```python
from build123d import *

# Parameters (mm, degrees)
SKETCH_W        = 70.25
SKETCH_H        = 49.7
PAD_DEPTH       = 7.1
SKETCH001_W     = 3.6
SKETCH001_H     = 9.8
SKETCH001_H_2   = 30.5
POCKET_DEPTH    = 0.9
SKETCH002_W     = 51.75
SKETCH002_H     = 5.3
PAD001_DEPTH    = 2.6
FILLET_R        = 1
SKETCH003_W     = 61.57
SKETCH003_H     = 44.62
PAD002_DEPTH    = 0.05
SKETCH004_R     = 1
POCKET001_DEPTH = 9.751


with BuildPart() as part:
    # Sketch → Pad (new body)
    with BuildSketch(Plane.XY):
        Rectangle(SKETCH_W, SKETCH_H)
    extrude(amount=PAD_DEPTH)

    # Sketch001 (on Face6 of Pad) → Pocket (cut)
    with BuildSketch(Plane.XY.offset(7.1)):
        with Locations((33.325, 19.95)):
            Rectangle(SKETCH001_W, SKETCH001_H)
        with Locations((33.325, -9.6)):
            Rectangle(SKETCH001_W, SKETCH001_H_2)
    extrude(amount=-POCKET_DEPTH, mode=Mode.SUBTRACT)

    # Sketch002 (on Face2 of Pocket) → Pad001 (join)
    with BuildSketch(Plane(origin=(0, 0, 0), x_dir=(1, 0, 0), z_dir=(0, 0, -1))):
        with Locations((-0.75, -22.2)):
            Rectangle(SKETCH002_W, SKETCH002_H)
    extrude(amount=PAD001_DEPTH)

    # Fillet
    fillet_edges = [part.edges().sort_by_distance(p)[0] for p in [
        (35.125, 10.35, 7.1),
    ]]
    fillet(fillet_edges, radius=FILLET_R)

    # Sketch003 (on Face8 of Fillet) → Pad002 (join)
    with BuildSketch(Plane.XY.offset(7.1)):
        with Locations((-1.8, 0)):
            Rectangle(SKETCH003_W, SKETCH003_H)
    extrude(amount=PAD002_DEPTH)

    # Sketch004 (on Face23 of Pad002) → Pocket001 (cut, through all)
    with BuildSketch(Plane.XY.offset(7.15)):
        Circle(SKETCH004_R)
    extrude(amount=-POCKET001_DEPTH, mode=Mode.SUBTRACT)


solid = part.part
```
Part model, mm, in its own coordinate system. A direction names the side the tool comes from. Round coordinates to 2 decimals unless told otherwise and drop trailing zeros. Loops run counter-clockwise (first coordinate to the right, second up) from the corner with the lowest first, then second, coordinate; pieces in that order, holes last. Notation, with made-up numbers: (-15, 58) -> (-4, 58) arc R30 cw to (-4, 93) -> close; hole circle Ø7 at (66.25, -31.5). An arc over 180 degrees is marked (long way). Use CSV: the item, a comma, the result in double quotes. Start each with the question number.
1) Cut at C-C, the plane x = 7.5. Write the cut outline in (y, z), plus the area to 3 significant figures.
2) Pull direction Y, two halves, no side cores. Call faces 1 (the flat face through (-35.125, 0, 4)), 2 (the cylindrical face through (0, -1, 4)), 3 (the flat face through (0, 24.85, 2)), 4 (the flat face through (-1, 19.55, -1)): +Y half, -Y half, draft (parallel to the pull), parting line (faces both ways), or undercut.
3) Which spindle directions (+Z, -Z, +X, -X, +Y, -Y) get a long thin tool onto all of the face, cutting with end or side? Do faces 5 (the flat face through (33, 20, 6.2)), 6 (the flat face through (25.125, 22, -1)), 7 (the flat face through (33, -9, 6.2)), 8 (the flat face through (-26.625, 22, -1)). Say none if no direction does.
4) Cut at D-D, the plane y = 8. Write the cut outline in (x, z) (3 decimals).
5) Cut at A-A, the plane y = 0. Write the cut outline in (x, z) (3 decimals).
6) Cut at B-B, the plane x = 0. Write the cut outline in (y, z).
7) Wall check: L1, parallel to Y at x = 0, z = 2.25; L2, parallel to Z at x = 7.5, y = -11; L3, parallel to Y at x = 14, z = -0.25. Give the ranges that are in metal, low to high. Write a range as [from, to].
8) Drop flat-ended pins along their axis: P1, Ø2, axis at x = 15, y = 11, coming from the -Z side; P2, Ø3, axis at x = 34, y = -6, coming from the +Z side; P3, Ø0.5, axis at y = -6.5, z = 6.5, coming from the +X side (3 decimals); P4, Ø0.7, axis at x = 32.5, z = 6.5, coming from the -Y side. Give the stop position or say it passes through.
Determined:
1,outline,"(-24.85, 0) -> (19.55, 0) -> (19.55, -2.6) -> (24.85, -2.6) -> (24.85, 7.1) -> (22.31, 7.1) -> (22.31, 7.15) -> (-22.31, 7.15) -> (-22.31, 7.1) -> (-24.85, 7.1) -> close"
1,area,"369 mm2"
2,face 1,"draft"
2,face 2,"undercut"
2,face 3,"+Y half"
2,face 4,"-Y half"
3,face 5,"+Z, +X, +Y"
3,face 6,"-Z, +X, +Y, -Y"
3,face 7,"+Z, +X, -Y"
3,face 8,"-Z, -X, +Y, -Y"
4,outline,"(-35.125, 0) -> (35.125, 0) -> (35.125, 6.1) arc R1 ccw to (34.125, 7.1) -> (28.985, 7.1) -> (28.985, 7.15) -> (-32.585, 7.15) -> (-32.585, 7.1) -> (-35.125, 7.1) -> close"
5,outline,"(-35.125, 0) -> (-1, 0) -> (-1, 7.15) -> (-32.585, 7.15) -> (-32.585, 7.1) -> (-35.125, 7.1) -> close; (1, 0) -> (35.125, 0) -> (35.125, 6.1) arc R1 ccw to (35.12, 6.2) -> (31.525, 6.2) -> (31.525, 7.1) -> (28.985, 7.1) -> (28.985, 7.15) -> (1, 7.15) -> close"
6,outline,"(-24.85, 0) -> (-1, 0) -> (-1, 7.15) -> (-22.31, 7.15) -> (-22.31, 7.1) -> (-24.85, 7.1) -> close; (1, 0) -> (19.55, 0) -> (19.55, -2.6) -> (24.85, -2.6) -> (24.85, 7.1) -> (22.31, 7.1) -> (22.31, 7.15) -> (1, 7.15) -> close"
7,L1,"y = [-24.85, -1], [1, 24.85]"
7,L2,"z = [0, 7.15]"
7,L3,"y = [19.55, 24.85]"
8,P1,"stops at z = 0"
8,P2,"stops at z = 6.2"
8,P3,"stops at x = 31.525"
8,P4,"stops at y = -24.85"
